from build123d import *

# Parameters (mm, degrees)
F0_R     = 44.45
F0_R_2   = 12.7
F2_DEPTH = 6.35


# Not quite as in the source:
# - a feature of the source that left no trace in its solid (it failed there, or was rolled back) is left out


with BuildPart() as f2:
    # F0 (on Top) → F2 (new body)
    with BuildSketch(Plane.XY):
        with BuildLine():
            ThreePointArc((46.13671875, -43.6308741946), (59.3475236203, -34.5646316236), (75.1176136364, -31.7315448688))
            ThreePointArc((75.1176136364, -31.7315448688), (107.95, 0), (75.1176136364, 31.7315448688))
            ThreePointArc((75.1176136364, 31.7315448688), (59.3475236203, 34.5646316236), (46.13671875, 43.6308741946))
            ThreePointArc((46.13671875, 43.6308741946), (0, 63.5), (-46.13671875, 43.6308741946))
            ThreePointArc((-46.13671875, 43.6308741946), (-59.3475236203, 34.5646316236), (-75.1176136364, 31.7315448688))
            ThreePointArc((-75.1176136364, 31.7315448688), (-107.95, 0), (-75.1176136364, -31.7315448688))
            ThreePointArc((-75.1176136364, -31.7315448688), (-59.3475236203, -34.5646316236), (-46.13671875, -43.6308741946))
            ThreePointArc((-46.13671875, -43.6308741946), (0, -63.5), (46.13671875, -43.6308741946))
        make_face()
        with BuildLine():
            ThreePointArc((-75.9357507288, 12.6972505812), (-66.7851626656, 9.0732013574), (-62.9715014577, 0))
            ThreePointArc((-62.9715014577, 0), (-66.7851626656, -9.0732013574), (-75.9357507288, -12.6972505812))
            ThreePointArc((-75.9357507288, -12.6972505812), (-88.9, 0), (-75.9357507288, 12.6972505812))
        make_face(mode=Mode.SUBTRACT)
        Circle(F0_R, mode=Mode.SUBTRACT)
        with Locations((76.2, 0)):
            Circle(F0_R_2, mode=Mode.SUBTRACT)
    extrude(amount=F2_DEPTH)


solid = f2.part
Can you work these out from the model? Positions are in its coordinate system, mm. A direction names the side the tool comes from. Give positions to 0.01 mm unless a question says otherwise; leave off trailing zeros. Loops run counter-clockwise (first coordinate to the right, second up) from the corner with the lowest first, then second, coordinate; pieces in that order, holes last. Notation, with made-up numbers: (-24, 40.5) -> (10, 40.5) arc R24 cw to (10, 71.5) -> close; hole circle Ø10 at (38, 8.5). An arc over 180 degrees is marked (long way). Use one line per item in the form item = value.
1) If we section it at B-B (y = -6): Please give me the cut outline in (x, z), plus the area to 3 significant figures.
Answers:
outline = (-107.38, 0) -> (-87.39, 0) -> (-87.39, 6.35) -> (-107.38, 6.35) -> close; (-64.48, 0) -> (-44.04, 0) -> (-44.04, 6.35) -> (-64.48, 6.35) -> close; (44.04, 0) -> (65.01, 0) -> (65.01, 6.35) -> (44.04, 6.35) -> close; (87.39, 0) -> (107.38, 0) -> (107.38, 6.35) -> (87.39, 6.35) -> close
area = 517 mm²
2) If we section it at C-C (y = 17): Please give me the cut outline in (x, z).
Answers:
outline = (-103.02, 0) -> (-41.07, 0) -> (-41.07, 6.35) -> (-103.02, 6.35) -> close; (41.07, 0) -> (103.02, 0) -> (103.02, 6.35) -> (41.07, 6.35) -> close
3) If we section it at D-D (z = 1): Please give me the cut outline in (x, y), plus the area to 3 significant figures.
Answers:
outline = (-75.12, -31.73) arc R38.1 cw to (-46.14, -43.63) arc R63.5 ccw to (46.14, -43.63) arc R38.1 cw to (75.12, -31.73) arc R31.75 ccw (long way) to (75.12, 31.73) arc R38.1 cw to (46.14, 43.63) arc R63.5 ccw to (-46.14, 43.63) arc R38.1 cw to (-75.12, 31.73) arc R31.75 ccw (long way) to start; hole (-75.94, -12.7) arc R12.7 ccw (long way) to (-75.94, 12.7) arc R12.7 ccw (long way) to start; hole circle Ø88.9 at (0, 0); hole circle Ø25.4 at (76.2, 0)
area = 10,700 mm²
4) If we section it at A-A (x = 0): Please give me the cut outline in (y, z), plus the area to 3 significant figures.
Answers:
outline = (-63.5, 0) -> (-44.45, 0) -> (-44.45, 6.35) -> (-63.5, 6.35) -> close; (44.45, 0) -> (63.5, 0) -> (63.5, 6.35) -> (44.45, 6.35) -> close
area = 242 mm²
5) I need wall thicknesses on line 1 along Y through (x, z) = (0, 4); line 2 along Y through (x, z) = (76.2, 2); line 3 along X through (y, z) = (-23, 5.75). Which ranges of each line are inside material? Lowest first, please.
Answers:
line_1 = -63.5 to -44.45, 44.45 to 63.5
line_2 = -31.75 to -12.7, 12.7 to 31.75
line_3 = -98.09 to -38.04, 38.04 to 98.09
6) Will these pins go through, and if not, where does the flat tip stop? pin 1 (3 mm diameter, centred on x = 65, z = 1, fed in from -Y); pin 2 (3 mm diameter, centred on x = -30.5, z = 0.5, fed in from -Y).
Answers:
pin_1 = -33.13
pin_2 = -56.49
7) For faces 1 (the face through (-88.897, -0.283, 3.131)), 2 (the face through (0.723, 63.496, 3.131)), which set-ups out of +Z, -Z, +X, -X, +Y, -Y let a thin tool reach every point of the face, with its end or its side?
Answers:
face_1 = +Z, -Z
face_2 = +Z, -Z, +Y
8) We'd pull the mould along Y, two halves only. Please class faces 3 (the face through (42.397, 13.352, 3.131)), 4 (the face through (46, 1, 0)), 5 (the face through (59.14, -34.65, 3.13)): released by +Y, released by -Y, zero draft, split by the parting line, or undercut.
Answers:
face_3 = undercut
face_4 = zero draft
face_5 = released by -Y
